Build history of the part. All positions in model axes, mm. A direction names the side the tool comes from. Round coordinates to 2 decimals unless told otherwise and drop trailing zeros. Order: outer loops, then holes, each group sorted by start corner. A loop starts at its lowest first (then second) coordinate and runs counter-clockwise, first axis right, second up. Notation, with made-up numbers: M 53.25,56.25 L 78.25,56.25 A22 ccw 78.25,94.25 Z; hole C 5,-3 d8. An arc over 180 degrees is marked long. One line per item, written item: value. Start each with the question number.
Item 1: Two-plate mould, pull along Y, no slides. Class faces 4 (the flat face through (0, 0, 1.588)), 5 (the cylindrical face through (-12.477, -12.378, 9.658)), 6 (the flat face through (-38.164, 0, 10)): +Y half, -Y half, draft (parallel to the pull), parting line (faces both ways), or undercut.
Item 2: Tool access for faces 1 (the flat face through (-26, -6.668, 10)), 2 (the flat face through (14.288, -7, 9)), 3 (the flat face through (-26, 6.668, 10)): list every direction of +Z, -Z, +X, -X, +Y, -Y with a clear straight run to the whole face (end or side of a thin tool).
Item 3: Band-saw the part on B-B, the plane x = -32. Write the cut outline in (y, z), then the cut area to 3 significant figures.
Item 4: Band-saw the part on A-A, the plane y = 0. Give the number of separate pieces and of enclosed holes in the cut face, then the cut area to 3 significant figures.
Item 5: Pin check, flat tips, straight feed: pin 1 (15 mm diameter, centred on x = -31.81, y = 0, fed in from +Z); pin 2 (5.5 mm diameter, centred on x = -28, z = 12, fed in from +Y); pin 3 (3 mm diameter, centred on x = 30.5, y = -2, fed in from -Z); pin 4 (1.5 mm diameter, centred on x = -30, z = 12.5, fed in from -Y). Stop position of each tip, or through.
Item 6: Probe L1, parallel to Z at x = 6, y = -1.5; L2, parallel to Y at x = 18, z = 1.25; L3, parallel to Y at x = -32.5, z = 10. List the from-to ranges inside material, lowest first.
```python
from build123d import *

# Parameters (mm, degrees)
SKETCH2_W           = 28.575
SKETCH2_H           = 28.575
BOSS_EXTRUDE2_DEPTH = 19.05
SKETCH1_R           = 13.335
CUT_EXTRUDE4_DEPTH  = 1.5875
FILLET2_R           = 6.35
SKETCH3_W           = 19.05
SKETCH3_H           = 13.335
BOSS_EXTRUDE3_DEPTH = 23.876
SKETCH4_R           = 3.175
CUT_EXTRUDE5_DEPTH  = 45.983195623
SKETCH6_R           = 4.7625
CUT_EXTRUDE6_DEPTH  = 6.35


with BuildPart() as part:
    # Sketch2 → Boss-Extrude2 (new body)
    with BuildSketch(Plane.XY):
        Rectangle(SKETCH2_W, SKETCH2_H)
    extrude(amount=BOSS_EXTRUDE2_DEPTH)

    # Sketch1 → Cut-Extrude4 (cut)
    with BuildSketch(Plane.XY):
        Circle(SKETCH1_R)
    extrude(amount=CUT_EXTRUDE4_DEPTH, mode=Mode.SUBTRACT)

    # Fillet2
    fillet2_edges = [part.edges().sort_by_distance(p)[0] for p in [
        (14.2875, -14.2875, 9.525),
        (-14.2875, -14.2875, 9.525),
        (-14.2875, 14.2875, 9.525),
        (14.2875, 14.2875, 9.525),
    ]]
    fillet(fillet2_edges, radius=FILLET2_R)

    # Sketch3 → Boss-Extrude3 (add)
    with BuildSketch(Plane(origin=(14.2875, 0, 0), x_dir=(0, 0, -1), z_dir=(1, 0, 0))):
        with Locations((-9.525, 0)):
            Rectangle(SKETCH3_W, SKETCH3_H)
    boss_extrude3 = extrude(amount=BOSS_EXTRUDE3_DEPTH)

    # Sketch4 → Cut-Extrude5 (cut, symmetric)
    with BuildSketch(Plane(origin=(0, 0, 0), x_dir=(-1, 0, 0), z_dir=(0, 0, -1))):
        with Locations((-31.8135, 0)):
            Circle(SKETCH4_R)
    cut_extrude5 = extrude(amount=CUT_EXTRUDE5_DEPTH, both=True, mode=Mode.SUBTRACT)

    # Sketch6 → Cut-Extrude6 (cut)
    with BuildSketch(Plane(origin=(0, 0, 0), x_dir=(-1, 0, 0), z_dir=(0, 0, -1))):
        with Locations((-31.8135, 0)):
            Circle(SKETCH6_R)
    cut_extrude6 = extrude(amount=-CUT_EXTRUDE6_DEPTH, mode=Mode.SUBTRACT)

    # Mirror1: Boss-Extrude3, Cut-Extrude5, Cut-Extrude6 across plane
    add(boss_extrude3.mirror(Plane(origin=(0, 0, 0), x_dir=(0, 0, 1), z_dir=(1, 0, 0))))
    add(cut_extrude5.mirror(Plane(origin=(0, 0, 0), x_dir=(0, 0, 1), z_dir=(1, 0, 0))), mode=Mode.SUBTRACT)
    add(cut_extrude6.mirror(Plane(origin=(0, 0, 0), x_dir=(0, 0, 1), z_dir=(1, 0, 0))), mode=Mode.SUBTRACT)


solid = part.part
```
Output:
1. face 4: undercut
1. face 5: -Y half
1. face 6: draft
2. face 1: +Z, -Z, -X, -Y
2. face 2: +Z, -Z, +X, -Y
2. face 3: +Z, -Z, -X, +Y
3. outline: M -6.67,0 L -4.76,0 L -4.76,6.35 L -3.17,6.35 L -3.17,19.05 L -6.67,19.05 Z; M 3.17,6.35 L 4.76,6.35 L 4.76,0 L 6.67,0 L 6.67,19.05 L 3.17,19.05 Z
3. area: 113 mm²
4. separate pieces: 3
4. enclosed holes: 0
4. area: 1,130 mm²
5. pin 1: stops at z = 19.05
5. pin 2: stops at y = 6.67
5. pin 3: stops at z = 6.35
5. pin 4: stops at y = -6.67
6. L1: z = 1.59 to 19.05
6. L2: y = -6.67 to 6.67
6. L3: y = -6.67 to -3.1, 3.1 to 6.67
